```python
from build123d import *

# Parameters (mm, degrees)
SKETCH_1_W          = 60
SKETCH_1_H          = 54
EXTRUDE_1_DEPTH     = 3
SKETCH_3_R          = 3
SKETCH_3_R_2        = 1.25
EXTRUDE_2_DEPTH     = 3
SKETCH_4_R          = 1.25
CUT_EXTRUDE_1_DEPTH = 3
CHAMFER_1_SIZE      = 2.5


with BuildPart() as part:
    # Эскиз1 → Бобышка-Вытянуть1 (new body)
    with BuildSketch(Plane(origin=(0, 0, 0), x_dir=(1, 0, 0), z_dir=(0, 1, 0))):
        with Locations((-1.465707965, -0.838495575)):
            Rectangle(SKETCH_1_W, SKETCH_1_H)
    extrude(amount=-EXTRUDE_1_DEPTH)

    # Эскиз3 → Бобышка-Вытянуть2 (add)
    with BuildSketch(Plane(origin=(0, 0, 0), x_dir=(1, 0, 0), z_dir=(0, 1, 0))):
        with Locations((-27.465707965, 17.161504425)):
            Circle(SKETCH_3_R)
        with Locations((-27.465707965, 17.161504425)):
            Circle(SKETCH_3_R_2, mode=Mode.SUBTRACT)
        with Locations((-27.465707965, -17.838495575)):
            Circle(SKETCH_3_R)
        with Locations((-27.465707965, -17.838495575)):
            Circle(SKETCH_3_R_2, mode=Mode.SUBTRACT)
        with Locations((-8.465707965, 17.161504425)):
            Circle(SKETCH_3_R)
        with Locations((-8.465707965, 17.161504425)):
            Circle(SKETCH_3_R_2, mode=Mode.SUBTRACT)
        with Locations((-8.465707965, -17.838495575)):
            Circle(SKETCH_3_R)
        with Locations((-8.465707965, -17.838495575)):
            Circle(SKETCH_3_R_2, mode=Mode.SUBTRACT)
        with Locations((5.534292035, -17.838495575)):
            Circle(SKETCH_3_R)
        with Locations((5.534292035, -17.838495575)):
            Circle(SKETCH_3_R_2, mode=Mode.SUBTRACT)
        with Locations((5.534292035, 17.161504425)):
            Circle(SKETCH_3_R)
        with Locations((5.534292035, 17.161504425)):
            Circle(SKETCH_3_R_2, mode=Mode.SUBTRACT)
        with Locations((24.534292035, -17.838495575)):
            Circle(SKETCH_3_R)
        with Locations((24.534292035, -17.838495575)):
            Circle(SKETCH_3_R_2, mode=Mode.SUBTRACT)
        with Locations((24.534292035, 17.161504425)):
            Circle(SKETCH_3_R)
        with Locations((24.534292035, 17.161504425)):
            Circle(SKETCH_3_R_2, mode=Mode.SUBTRACT)
    extrude(amount=EXTRUDE_2_DEPTH)

    # Эскиз4 → Вырез-Вытянуть1 (cut)
    with BuildSketch(Plane(origin=(0, 0, 0), x_dir=(1, 0, 0), z_dir=(0, 1, 0))):
        with Locations((-17.965707965, -0.838495575)):
            Circle(SKETCH_4_R)
        with Locations((15.034292035, -0.838495575)):
            Circle(SKETCH_4_R)
    extrude(amount=-CUT_EXTRUDE_1_DEPTH, mode=Mode.SUBTRACT)

    # Фаска1
    chamfer_1_edges = [part.edges().sort_by_distance(p)[0] for p in [
        (-19.215707965, 0, 0.838495575),
        (13.784292035, 0, 0.838495575),
    ]]
    chamfer(chamfer_1_edges, length=CHAMFER_1_SIZE)


solid = part.part
```
The model under review builds one solid part; all positions refer to its coordinate system, in mm. A direction names the side the tool comes from. Give positions to 0.01 mm unless a question says otherwise; leave off trailing zeros. Loops run counter-clockwise (first coordinate to the right, second up) from the corner with the lowest first, then second, coordinate; pieces in that order, holes last. Notation, with made-up numbers: (-31, 27.5) -> (-14, 27.5) arc R16 cw to (-14, 48.5) -> close; hole circle Ø3 at (88, 49.5). An arc over 180 degrees is marked (long way). Use CSV: the item, a comma, the result in double quotes.
1. The part is to be moulded in two halves that separate along Z. For faces 3 (the face through (-31.466, -1, 1)), 4 (the face through (-28.458, 1.479, -16.401)), say which applies: +Z half, -Z half, draft (parallel to the pull), parting line (faces both ways), or undercut.
Result:
face 3,"draft"
face 4,"undercut"
2. Consider section C-C, the plane x = -1. Write out the cut boundary in (y, z), then the cut area to 3 significant figures.
Result:
outline,"(-3, -26.16) -> (0, -26.16) -> (0, 27.84) -> (-3, 27.84) -> close"
area,"162 mm²"
3. Consider section A-A, the plane y = 0.75. Count the separate pieces of the cut face and the enclosed holes in it, then the cut area to 3 significant figures.
Result:
separate pieces,"8"
enclosed holes,"8"
area,"187 mm²"
4. Consider section D-D, the plane z = 8.5. Write out the cut boundary in (x, y), then the cut area to 3 significant figures.
Result:
outline,"(-31.47, -3) -> (28.53, -3) -> (28.53, 0) -> (-31.47, 0) -> close"
area,"180 mm²"
5. To check wall thickness, follow probe 1 along Z at (x, y) = (-27.5, 1.35); probe 2 along Z at (x, y) = (-7.5, 0.05); probe 3 along Z at (x, y) = (22.5, 0.7). State the ranges of each line that lie inside material, in increasing order. Write a range as from..to.
Result:
probe 1,"z = -20.16..-18.41, -15.91..-14.16, 14.84..16.59, 19.09..20.84"
probe 2,"z = -20..-17.96, -16.37..-14.32, 15..17.04, 18.63..20.68"
probe 3,"z = -19.37..-14.96, 15.63..20.04"
6. Machinability: for faces 1 (the face through (-27, 0, -17)), 2 (the face through (-2, -3, 0)), which of the approach directions +Z, -Z, +X, -X, +Y, -Y give a long, thin tool a straight path to every point of the face, cutting with its end or side? Answer none if there is none.
Result:
face 1,"+Y"
face 2,"+Z, -Z, +X, -X, -Y"
7. Consider section B-B, the plane z = 20. Write out the cut boundary in (x, y).
Result:
outline,"(-31.47, -3) -> (28.53, -3) -> (28.53, 0) -> (26.61, 0) -> (26.61, 3) -> (22.45, 3) -> (22.45, 0) -> (7.61, 0) -> (7.61, 3) -> (3.45, 3) -> (3.45, 0) -> (-6.39, 0) -> (-6.39, 3) -> (-10.55, 3) -> (-10.55, 0) -> (-25.39, 0) -> (-25.39, 3) -> (-29.55, 3) -> (-29.55, 0) -> (-31.47, 0) -> close"
8. For P1, Ø1.5, axis at x = -17.97, z = 0.84, coming from the -Y side; P2, Ø0.8, axis at x = 24.5, z = -17, coming from the +Y side, all flat-tipped, find the tip position at first contact; note any pin that passes through.
Result:
P1,"passes through"
P2,"stops at y = 0"
